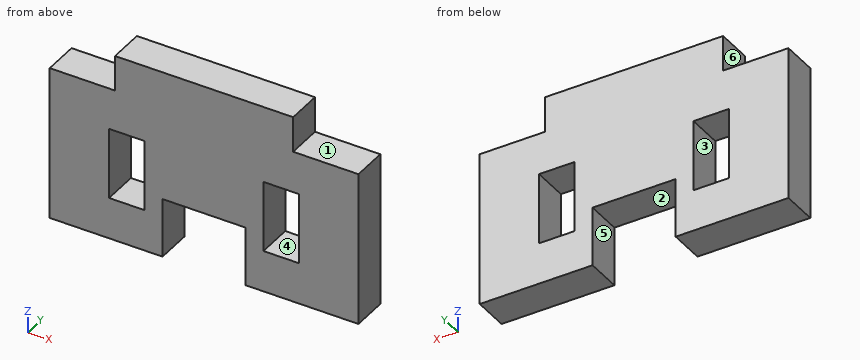
```python
from build123d import *

# Parameters (mm, degrees)
SALIENTE_EXTRUIR1_DEPTH = 3


with BuildPart() as part:
    # Croquis1 → Saliente-Extruir1 (new body)
    with BuildSketch(Plane(origin=(0, 0, 0), x_dir=(1, 0, 0), z_dir=(0, 1, 0))):
        Polygon((0, 0), (15, 0), (15, 3), (20.5, 3), (20.5, 16), (11, 16), (11, 11), (7.5, 11), (4, 11), (4, 16), (-5.5, 16), (-5.5, 3), (0, 3), align=None)
        Polygon((1, 12.5), (2.5, 12.5), (2.5, 6.5), (-0.5, 6.5), (-0.5, 12.5), align=None, mode=Mode.SUBTRACT)
        Polygon((12.5, 6.5), (15.5, 6.5), (15.5, 12.5), (14, 12.5), (12.5, 12.5), align=None, mode=Mode.SUBTRACT)
    extrude(amount=SALIENTE_EXTRUIR1_DEPTH)


solid = part.part
```
Here's how the part is built. I have some questions about the finished solid (model axes, mm). Face numbers are marked on the shaded views. A direction names the side the tool comes from. Coordinates: 2 decimals unless noted, no trailing zeros. Loops run counter-clockwise (first coordinate to the right, second up) from the corner with the lowest first, then second, coordinate; pieces in that order, holes last. Notation, with made-up numbers: (14.25, -17) - (48.25, -17) arc R23 cw to (48.25, 3) - close; hole circle Ø1 at (-0.75, 30). An arc over 180 degrees is marked (long way). Answer as CSV lines item,"result".
Q1. For the marked faces 4, 5 and 6, which set-ups out of +Z, -Z, +X, -X, +Y, -Y let a thin tool reach every point of the face, with its end or its side?
Response:
face 4,"+Y, -Y"
face 5,"-Z, +Y, -Y"
face 6,"+Z, -X, +Y, -Y"
Q2. For pin 1 (0.9 mm diameter, centred on x = 9, y = 1.5, fed in from -Z); pin 2 (1.5 mm diameter, centred on x = 1.5, y = 1.5, fed in from +Z); pin 3 (0.9 mm diameter, centred on x = 17.5, y = 1.5, fed in from +Z); pin 4 (0.9 mm diameter, centred on y = 1.5, z = -1, fed in from +X), each with a flat end and sliding along its axis, tell me the tip position at first contact or that it passes through.
Response:
pin 1,"z = -11"
pin 2,"z = 0"
pin 3,"z = -3"
pin 4,"x = 15"
Q3. If I drill on L1, parallel to X at y = 2.9, z = -9; L2, parallel to Z at x = 14.25, y = 2.65; L3, parallel to X at y = 1, z = -14.75, over which ranges is the centre line in solid material (lowest first)? Write a range as [from, to].
Response:
L1,"[-5.5, -0.5], [2.5, 12.5], [15.5, 20.5]"
L2,"[-16, -12.5], [-6.5, 0]"
L3,"[-5.5, 4], [11, 20.5]"
Q4. If we section it at C-C, the plane x = -1.5: Write out the boundary of the cut face in (y, z).
Response:
outline,"(0, -16) - (3, -16) - (3, -3) - (0, -3) - close"
Q5. If we section it at A-A, the plane y = 0.45: Write out the boundary of the cut face in (x, z), and give its area (3 significant figures).
Response:
outline,"(-5.5, -16) - (4, -16) - (4, -11) - (11, -11) - (11, -16) - (20.5, -16) - (20.5, -3) - (15, -3) - (15, 0) - (0, 0) - (0, -3) - (-5.5, -3) - close; hole (-0.5, -12.5) - (2.5, -12.5) - (2.5, -6.5) - (-0.5, -6.5) - close; hole (12.5, -12.5) - (15.5, -12.5) - (15.5, -6.5) - (12.5, -6.5) - close"
area,"312 mm2"
Q6. If we section it at B-B, the plane z = -7: Write out the boundary of the cut face in (x, y), and give its area (3 significant figures).
Response:
outline,"(-5.5, 0) - (-0.5, 0) - (-0.5, 3) - (-5.5, 3) - close; (2.5, 0) - (12.5, 0) - (12.5, 3) - (2.5, 3) - close; (15.5, 0) - (20.5, 0) - (20.5, 3) - (15.5, 3) - close"
area,"60.0 mm2"
Q7. If we section it at D-D, the plane z = -1.75: Write out the boundary of the cut face in (x, y), and give its area (3 significant figures).
Response:
outline,"(0, 0) - (15, 0) - (15, 3) - (0, 3) - close"
area,"45.0 mm2"
Q8. We'd pull the mould along Z, two halves only. Please class the marked faces 1, 2 and 3: pulls with the +Z half, pulls with the -Z half, needs draft (parallel to the pull), parting line crosses it, or undercut.
Response:
face 1,"pulls with the +Z half"
face 2,"pulls with the -Z half"
face 3,"undercut"
